For this review, use the dimensioned drawing (mm, ordinates from the lowest corner) and the shaded views. A direction names the side the tool comes from. Give positions to 0.01 mm unless a question says otherwise; leave off trailing zeros. Order: outer loops, then holes, each group sorted by start corner. A loop starts at its lowest first (then second) coordinate and runs counter-clockwise, first axis right, second up. Notation, with made-up numbers: (40, 59) - (52, 59) arc R32 cw to (52, 95) - close; hole circle Ø9 at (-36.75, 57). An arc over 180 degrees is marked (long way). Use a Markdown table: item, result. Add a question column.
1) We need section D-D on z = 0.5. Write out the cut boundary in (x, y) (1 decimal).
2) We need section C-C on x = 15.5. Write out the cut boundary in (y, z) (1 decimal).
3) Machinability: for the marked faces 1 and 2, which of the approach directions +Z, -Z, +X, -X, +Y, -Y give a long, thin tool a straight path to every point of the face, cutting with its end or side? Answer none if there is none.
4) Mouldability with a two-part tool opening along Y and no side actions: class the marked faces 3, 4 and 5 as released by +Y, released by -Y, zero draft, split by the parting line, or undercut.
5) We need section A-A on z = 3.25. Write out the cut boundary in (x, y) (1 decimal).
6) Wall thickness on L1, parallel to Y at x = 18, z = 1 (1 decimal); L2, parallel to X at y = 18, z = 3.25 (1 decimal); L3, parallel to Y at x = 11, z = 2.5 (1 decimal): over which ranges is each line inside the solid? List them lowest first.
7) Clearance check with flat-ended pins moving along their axes: P1, Ø3.5, axis at y = 13.5, z = 3.5, coming from the +X side; P2, Ø2, axis at x = 5, z = 6.5, coming from the -Y side; P3, Ø1, axis at x = 24, z = 1, coming from the +Y side (1 decimal). State where each tip first meets the part, or that it passes through.
8) We need section B-B on y = 20.5. Write out the cut boundary in (x, z) (1 decimal).
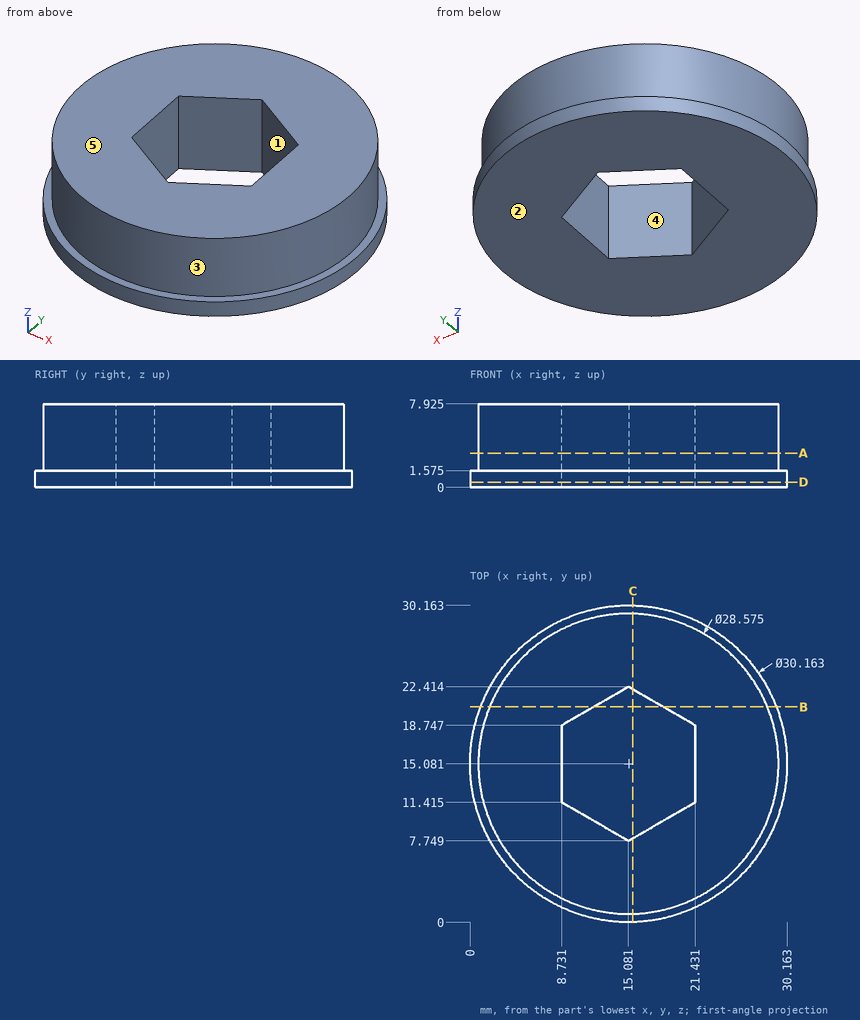
Checked values:
| question | item | result |
|---|---|---|
| 1 | outline | circle Ø30.2 at (15.1, 15.1); hole (8.7, 11.4) - (15.1, 7.7) - (21.4, 11.4) - (21.4, 18.7) - (15.1, 22.4) - (8.7, 18.7) - close |
| 2 | outline | (0, 0) - (8, 0) - (8, 7.9) - (0.8, 7.9) - (0.8, 1.6) - (0, 1.6) - close; (22.2, 0) - (30.2, 0) - (30.2, 1.6) - (29.4, 1.6) - (29.4, 7.9) - (22.2, 7.9) - close |
| 3 | face 1 | +Z, -Z |
| 3 | face 2 | -Z, +X, -X, +Y, -Y |
| 4 | face 3 | split by the parting line |
| 4 | face 4 | undercut |
| 4 | face 5 | zero draft |
| 5 | outline | circle Ø28.6 at (15.1, 15.1); hole (8.7, 11.4) - (15.1, 7.7) - (21.4, 11.4) - (21.4, 18.7) - (15.1, 22.4) - (8.7, 18.7) - close |
| 6 | L1 | 0.3 to 9.4, 20.7 to 29.9 |
| 6 | L2 | 1.1 to 8.7, 21.4 to 29.1 |
| 6 | L3 | 1.4 to 10.1, 20.1 to 28.8 |
| 7 | P1 | x = 29.37 |
| 7 | P2 | y = 4.05 |
| 7 | P3 | y = 27.6 |
| 8 | outline | (1, 0) - (11.8, 0) - (11.8, 7.9) - (1.9, 7.9) - (1.9, 1.6) - (1, 1.6) - close; (18.4, 0) - (29.2, 0) - (29.2, 1.6) - (28.3, 1.6) - (28.3, 7.9) - (18.4, 7.9) - close |
